```python
from build123d import *

# Parameters (mm, degrees)
SKETCH_R  = 20
PAD_DEPTH = 1


with BuildPart() as sphere:
    # Sphere → Sphere (revolve)
    with BuildSketch(Plane(origin=(0, 0, 7), x_dir=(1, 0, 0), z_dir=(0, -1, 0))):
        with BuildLine():
            ThreePointArc((0, -20), (20, 0), (0, 20))
            Line((0, 20), (0, -20))
        make_face()
    revolve(axis=Axis((0, 0, 7), (0, 0, 1)))


with BuildPart() as cut:
    # Sketch → Pad (new body)
    with BuildSketch(Plane.XY):
        Circle(SKETCH_R)
    extrude(amount=PAD_DEPTH)

    # Cut: cut Sphere
    add(sphere.part, mode=Mode.SUBTRACT)


solid = cut.part
```
The listing builds one solid part. Answer for the finished solid, in the listing's coordinates (mm). Round coordinates to 2 decimals unless told otherwise and drop trailing zeros. Loops run counter-clockwise (first coordinate to the right, second up) from the corner with the lowest first, then second, coordinate; pieces in that order, holes last.
Q1. Section B-B, the plane y = 13 is taken. Determine the outline of the cut face in (x, z).
Q2. Section C-C, the plane z = 0.7 is taken. Determine the outline of the cut face in (x, y), then the cut area to 3 significant figures.
Q3. Given pin 1 Ø1.5 at (x, y) = (-10, -12.5) entering from +Z, flat-ended and moving along its own axis, determine where the tip first touches the part or whether it passes through.
Q4. Section A-A, the plane x = -6 is taken. Determine the outline of the cut face in (y, z).
Q5. Find the intervals of material crossed by line 1 (X direction, y = -1.5, z = 0.35); line 2 (Y direction, x = 17, z = 0.25); line 3 (X direction, y = 11, z = 0.4), in increasing order.
Completed:
1. outline: (-15.2, 0) - (-13.49, 0) arc R15.2 cw to (-13.96, 1) - (-15.2, 1) - close; (13.49, 0) - (15.2, 0) - (15.2, 1) - (13.96, 1) arc R15.2 cw to start
2. outline: circle Ø40 at (0, 0); hole circle Ø37.96 at (0, 0)
2. area: 125 mm2
3. pin 1: passes through
4. outline: (-19.08, 0) - (-17.75, 0) arc R19.08 cw to (-18.11, 1) - (-19.08, 1) - close; (17.75, 0) - (19.08, 0) - (19.08, 1) - (18.11, 1) arc R19.08 cw to start
5. line 1: x = -19.94 to -18.8, 18.8 to 19.94
5. line 2: y = -10.54 to -8.09, 8.09 to 10.54
5. line 3: x = -16.7 to -15.34, 15.34 to 16.7
